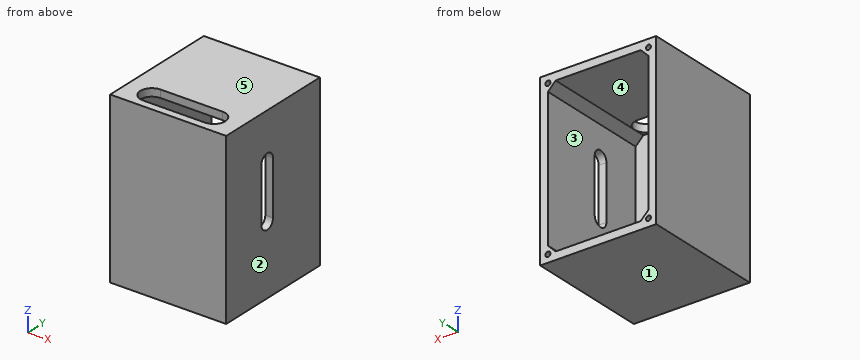
Autodesk Inventor part; units mm, degrees
ref_plane "YZ Plane" through (0, 0, 0) normal (1, 0, 0) x (0, 1, 0)
ref_plane "XZ Plane" through (0, 0, 0) normal (0, 1, 0) x (-1, 0, 0)
ref_plane "XY Plane" through (0, 0, 0) normal (0, 0, 1) x (1, 0, 0)
sketch "Sketch1" plane through (0, 0, 0) normal (0, 1, 0) x (-1, 0, 0)
  line L0 (32.5, 50) -> (-32.5, 50)
  line L1 (-32.5, 50) -> (-32.5, -50)
  line L2 (-32.5, -50) -> (32.5, -50)
  line L3 (32.5, -50) -> (32.5, 50)
  line L4 (32.5, 50) -> (-32.5, -50) construction
  line L5 (-32.5, 50) -> (32.5, -50) construction
  line L6 (37.5, -55) -> (-37.5, -55)
  line L7 (-37.5, -55) -> (-37.5, 55)
  line L8 (-37.5, 55) -> (37.5, 55)
  line L9 (37.5, 55) -> (37.5, -55)
  line L10 (-32.5, 45) -> (-27.5, 50)
  line L11 (-32.5, 45) -> (-25.4289, 45) construction
  line L12 (0, 55) -> (0, -55) construction
  line L13 (-37.5, 0) -> (37.5, 0) construction
  line L14 (32.5, 45) -> (27.5, 50)
  line L15 (-32.5, -45) -> (-27.5, -50)
  line L16 (32.5, -45) -> (27.5, -50)
  point P0 (0, 0)
  dimension "d0" = 100
  dimension "d1" = 65
  dimension "d2" = 5
  dimension "d29" = 45
  dimension "d30" = 5
extrude "Extrusion1" add sketch "Sketch1" along normal blind 80 contours L3 L14 L0 | L10 L1 L0 | L3 L2 L16 | L15 L2 L1 | L6 L7 L8 L9
extrude "Extrusion2" add sketch "Sketch1" along normal blind 5 contours L3 L14 L0 | L14 L3 L16 L2 L15 L1 L10 L0 | L10 L1 L0 | L3 L2 L16 | L15 L2 L1
sketch "Sketch3" plane through (37.5, 0, 55) normal (1, 0, 0) x (0, 0, -1)
  line L0 (30, 40) -> (65, 40) construction
  line L1 (65, 40) -> (65, 30) construction
  line L2 (65, 30) -> (30, 30) construction
  line L3 (30, 30) -> (30, 40) construction
  line L4 (30, 40) -> (65, 30) construction
  line L5 (65, 40) -> (30, 30) construction
  line L6 (0, 0) -> (110, 0)
  line L7 (0, 0) -> (0, 80)
  line L8 (30, 35) -> (65, 35) construction
  line L9 (30, 30) -> (65, 30)
  line L10 (65, 40) -> (30, 40)
  arc A0 (30, 40) -> (30, 30) centre (30, 35) ccw
  arc A1 (65, 30) -> (65, 40) centre (65, 35) ccw
  point P0 (55, 0)
  point P1 (47.5, 35)
  point P2 (47.5, 40)
  dimension "d12" = 30
  dimension "d13" = 10
  dimension "d14" = 30
  dimension "d15" = 35
extrude "Extrusion4" cut sketch "Sketch3" against normal up to next
sketch "Sketch4" plane through (0, 80, 0) normal (0, 1, 0) x (1, 0, 0)
  line L0 (-37.5, -55) -> (37.5, -55)
  line L1 (37.5, -55) -> (37.5, 55)
  line L2 (37.5, 55) -> (-37.5, 55)
  line L3 (-37.5, 55) -> (-37.5, -55)
  point P0 (0, 0)
  point P1 (-32.5, -50)
  point P2 (-32.5, 50)
  point P3 (32.5, 50)
  point P4 (32.5, -50)
  dimension "d25" = 5
  dimension "d26" = 5
  dimension "d27" = 5
  dimension "d28" = 5
hole "Hole1" at (-32.5, 80, 50) at (-32.5, 80, -50) at (32.5, 80, -50) at (32.5, 80, 50) direction (0, -1, 0) diameter 3.2 depth 6
sketch "Sketch5" plane through (-37.5, 0, 55) normal (0, 0, 1) x (1, 0, 0)
  line L0 (65, 5) -> (10, 5)
  line L1 (17.5, 12.5) -> (57.5, 12.5) construction
  line L2 (17.5, 20) -> (57.5, 20)
  line L3 (57.5, 5) -> (17.5, 5)
  arc A0 (17.5, 20) -> (17.5, 5) centre (17.5, 12.5) ccw
  arc A1 (57.5, 5) -> (57.5, 20) centre (57.5, 12.5) ccw
  line L4 (10, 5) -> (10, 80)
  line L5 (65, 5) -> (65, 80)
  point P0 (37.5, 0)
  point P1 (37.5, 12.5)
  point P2 (37.5, 5)
  point P3 (10, 12.5)
  point P4 (65, 12.5)
  dimension "d31" = 15
extrude "Extrusion5" cut sketch "Sketch5" against normal up to next contours L0 A0 L2 A1
properties part number "DAQ_Housing_V1"
The listing builds one solid part. Answer for the finished solid, in the listing's coordinates (mm). Face numbers are marked on the shaded views. A direction names the side the tool comes from. Give positions to 0.01 mm unless a question says otherwise; leave off trailing zeros. Write each loop counter-clockwise with the first axis right and the second up, starting at its lowest first coordinate (ties: lowest second). Pieces come first, ordered by that corner, then holes. Notation, with made-up numbers: (3, 30.25) - (18, 30.25) arc R25 cw to (18, 68.25) - close; hole circle Ø5 at (-20, -2.5). An arc over 180 degrees is marked (long way). Use one line per item in the form item = value. Start each with the question number.
1) The mould has two halves that part along Z. Classify the marked faces 1, 2 and 3: pulls with the +Z half, pulls with the -Z half, needs draft (parallel to the pull), parting line crosses it, or undercut.
2) Find section C-C on y = 71.5. Determine the outline of the cut face in (x, z), plus the area to 3 significant figures.
3) Find section A-A on z = 11. Determine the outline of the cut face in (x, y), plus the area to 4 significant figures.
4) Find section D-D on x = 29. Determine the outline of the cut face in (y, z).
5) Find section B-B on x = -12. Determine the outline of the cut face in (y, z).
6) Consider line 1 along Z through (x, y) = (11.5, 44.5); line 2 along X through (y, z) = (55, -28.5); line 3 along Y through (x, z) = (-31, 30.5). Determine where each line is inside the solid, lowest interval first. Write a range as from..to.
7) A tool of negligible diameter and unlimited length cuts with its end or side. For the marked faces 4 and 5, from which of +Z, -Z, +X, -X, +Y, -Y can it reach the whole face along a straight path? Write none if from no direction.
8) Flat-ended cylindrical pins translate along their axes: pin 1 Ø1.5 at (x, z) = (23.5, 0) entering from +Y; pin 2 Ø1 at (x, z) = (33.5, -50) entering from +Y. Find the tip coordinate at first contact, or state that the pin passes through.
Geometry results:
q1.face_1 = pulls with the -Z half
q1.face_2 = needs draft
q1.face_3 = undercut
q2.outline = (-37.5, -55) - (37.5, -55) - (37.5, 55) - (-37.5, 55) - close; hole (-32.5, -45) - (-27.5, -50) - (27.5, -50) - (32.5, -45) - (32.5, 45) - (27.5, 50) - (-27.5, 50) - (-32.5, 45) - close
q2.area = 1,800 mm2
q3.outline = (-37.5, 0) - (37.5, 0) - (37.5, 30) - (32.5, 30) - (32.5, 5) - (-32.5, 5) - (-32.5, 80) - (-37.5, 80) - close; (32.5, 40) - (37.5, 40) - (37.5, 80) - (32.5, 80) - close
q3.area = 1,075 mm2
q4.outline = (0, -55) - (80, -55) - (80, -48.5) - (5, -48.5) - (5, 48.5) - (80, 48.5) - (80, 55) - (0, 55) - close
q5.outline = (0, -55) - (80, -55) - (80, -50) - (5, -50) - (5, 55) - (0, 55) - close; (20, 50) - (80, 50) - (80, 55) - (20, 55) - close
q6.line_1 = -55..-50, 50..55
q6.line_2 = -37.5..-32.5, 32.5..37.5
q6.line_3 = 0..5
q7.face_4 = +Y
q7.face_5 = +Z, +X, -X, +Y, -Y
q8.pin_1 = 5
q8.pin_2 = 74
